Here's the drawing with two shaded views (mm, measured from the low corner). I have some questions. A direction names the side the tool comes from. Give positions to 0.01 mm unless a question says otherwise; leave off trailing zeros. Write each loop counter-clockwise with the first axis right and the second up, starting at its lowest first coordinate (ties: lowest second). Pieces come first, ordered by that corner, then holes.
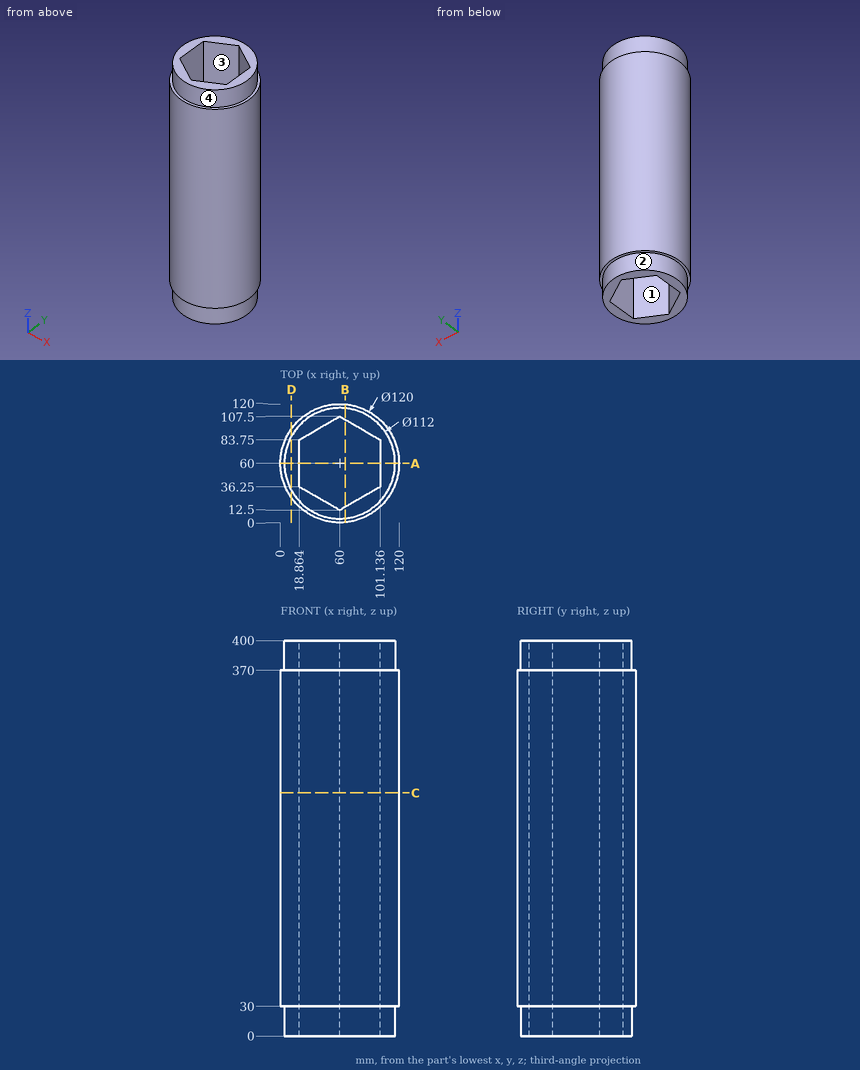
(1) Imagine slicing it at D-D, the plane x = 11. Write out the boundary of the cut face in (y, z), plus the area to 3 significant figures.
Returned:
outline: (25.37, 30) - (32.89, 30) - (32.89, 0) - (87.11, 0) - (87.11, 30) - (94.63, 30) - (94.63, 370) - (87.11, 370) - (87.11, 400) - (32.89, 400) - (32.89, 370) - (25.37, 370) - close
area: 26,800 mm2
(2) If we mould it in two halves opening along Y, with no side actions, what happens to the marked faces 3 and 4? For each: +Y half, -Y half, draft (parallel to the pull), parting line (faces both ways), or undercut.
Returned:
face 3: undercut
face 4: parting line
(3) Will these pins go through, and if not, where does the flat tip stop? P1, Ø5, axis at y = 97.5, z = 95, coming from the +X side; P2, Ø2, axis at x = 84.5, z = 311, coming from the -Y side; P3, Ø6, axis at x = 13.5, z = 311.5, coming from the -Y side (1 decimal).
Returned:
P1: stops at x = 108.73
P2: stops at y = 4.79
P3: stops at y = 18.7
(4) For the marked faces 1 and 2, which set-ups out of +Z, -Z, +X, -X, +Y, -Y let a thin tool reach every point of the face, with its end or its side?
Returned:
face 1: +Z, -Z
face 2: -Z
(5) Imagine slicing it at C-C, the plane z = 246. Write out the boundary of the cut face in (x, y).
Returned:
outline: circle Ø120 at (60, 60); hole (18.86, 36.25) - (60, 12.5) - (101.14, 36.25) - (101.14, 83.75) - (60, 107.5) - (18.86, 83.75) - close
(6) If I drill on L1, parallel to Y at x = 60, z = 311; L2, parallel to Z at x = 113, y = 83; L3, parallel to Y at x = 38.5, z = 78.5 (1 decimal), over which ranges is the centre line in solid material (lowest first)?
Returned:
L1: y = 0 to 12.5, 107.5 to 120
L2: z = 30 to 370
L3: y = 4 to 24.9, 95.1 to 116
(7) Imagine slicing it at A-A, the plane y = 60. Write out the boundary of the cut face in (x, z), plus the area to 3 significant figures.
Returned:
outline: (0, 30) - (4, 30) - (4, 0) - (18.86, 0) - (18.86, 400) - (4, 400) - (4, 370) - (0, 370) - close; (101.14, 0) - (116, 0) - (116, 30) - (120, 30) - (120, 370) - (116, 370) - (116, 400) - (101.14, 400) - close
area: 14,600 mm2
(8) Imagine slicing it at B-B, the plane x = 65.5. Write out the boundary of the cut face in (y, z), plus the area to 3 significant figures.
Returned:
outline: (0.25, 30) - (4.27, 30) - (4.27, 0) - (15.68, 0) - (15.68, 400) - (4.27, 400) - (4.27, 370) - (0.25, 370) - close; (104.32, 0) - (115.73, 0) - (115.73, 30) - (119.75, 30) - (119.75, 370) - (115.73, 370) - (115.73, 400) - (104.32, 400) - close
area: 11,900 mm2
